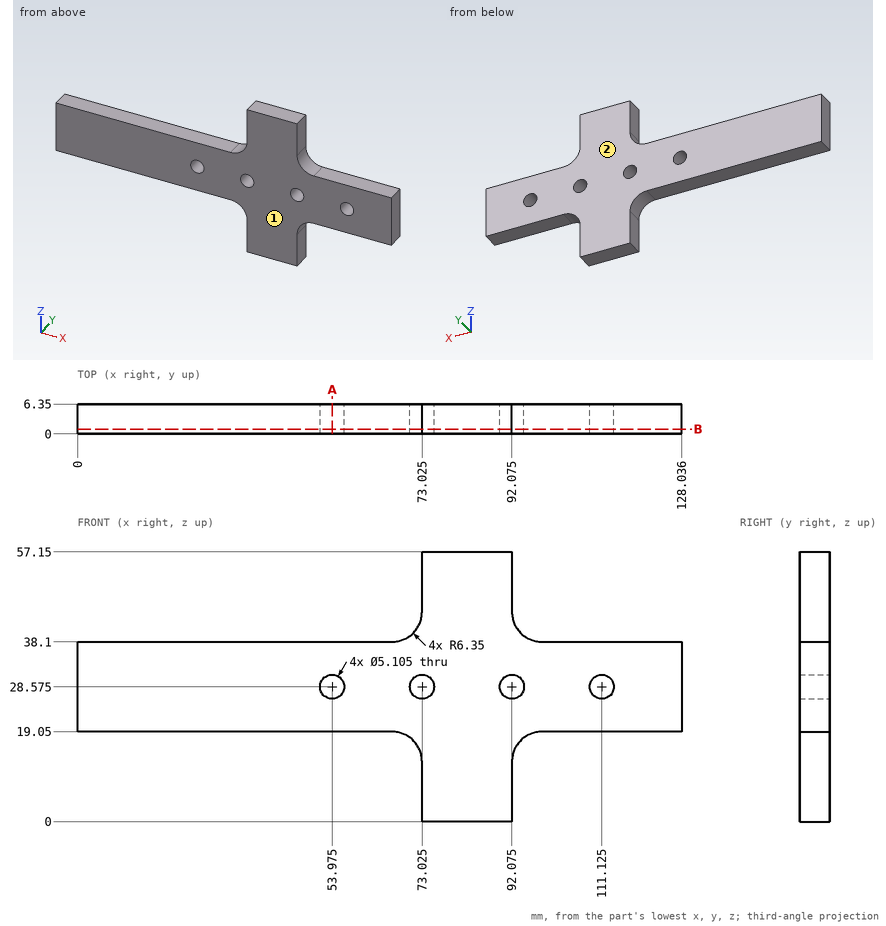
For this review, use the dimensioned drawing (mm, ordinates from the lowest corner) and the shaded views. Coordinates: 2 decimals unless noted, no trailing zeros. Order: outer loops, then holes, each group sorted by start corner. A loop starts at its lowest first (then second) coordinate and runs counter-clockwise, first axis right, second up. Notation, with made-up numbers: (79, -36) - (103, -36) arc R28 cw to (103, 2) - close; hole circle Ø10 at (12.25, 67). An arc over 180 degrees is marked (long way). Answer in a Markdown table with one row per item.
(1) Wall thickness on line 1 along X through (y, z) = (6, 26.5) (1 decimal); line 2 along X through (y, z) = (5.5, 29.5) (1 decimal); line 3 along Z through (x, y) = (11.5, 4.75): over which ranges is each line inside the solid? List them lowest first. Write a range as from..to.
Checked values:
| item | result |
|---|---|
| line 1 | 0..52.5, 55.5..71.5, 74.5..90.6, 93.6..109.6, 112.6..128 |
| line 2 | 0..51.6, 56.4..70.6, 75.4..89.7, 94.5..108.7, 113.5..128 |
| line 3 | 19.05..38.1 |
(2) Clearance check with flat-ended pins moving along their axes: pin 1 (1.9 mm diameter, centred on y = 2, z = 51, fed in from +X) (1 decimal); pin 2 (2 mm diameter, centred on x = 71.5, y = 5, fed in from +Z) (1 decimal); pin 3 (4 mm diameter, centred on x = 53.975, z = 28.575, fed in from -Y); pin 4 (1.9 mm diameter, centred on y = 4.5, z = 3.5, fed in from -X) (1 decimal). State where each tip first meets the part, or that it passes through.
Checked values:
| item | result |
|---|---|
| pin 1 | x = 92.1 |
| pin 2 | z = 41.9 |
| pin 3 | through |
| pin 4 | x = 73 |
(3) Consider section B-B on y = 1. Give the number of separate pieces and of enclosed holes in the cut face, plus the area to 3 significant figures.
Checked values:
| item | result |
|---|---|
| separate pieces | 1 |
| enclosed holes | 4 |
| area | 3,120 mm^2 |
(4) The part is to be moulded in two halves that separate along Y. For the marked faces 1 and 2, say which applies: released by +Y, released by -Y, zero draft, split by the parting line, or undercut.
Checked values:
| item | result |
|---|---|
| face 1 | released by -Y |
| face 2 | released by +Y |
(5) Consider section A-A on x = 54. State the section outline as (y, z) points.
Checked values:
| item | result |
|---|---|
| outline | (0, 19.05) - (6.35, 19.05) - (6.35, 26.02) - (0, 26.02) - close; (0, 31.13) - (6.35, 31.13) - (6.35, 38.1) - (0, 38.1) - close |
